```python
from build123d import *
from build123d.topology import SkipClean

# Parameters (mm, degrees)
SWEEP_2_DEPTH        = 3
SKETCH_15_W          = 3
SKETCH_15_H          = 8
SKETCH_17_W          = 3
SKETCH_17_H          = 8
REVOLVE_1_ANGLE      = 60
SKETCH_20_R          = 26.546275206
EXTRUDE_1_DEPTH      = 3
SKETCH_21_R          = 12.5
CUT_EXTRUDE_1_DEPTH  = 10
CUT_EXTRUDE_2_REACH  = 67.765
SKETCH_22_R          = 17
EXTRUDE_START        = 22
SKETCH_23_R          = 16.5
SKETCH_23_R_2        = 12.5
EXTRUDE_2_DEPTH      = 22
SKETCH_24_R          = 70.041464106
CUT_EXTRUDE_3_DEPTH  = 10
SKETCH_27_R          = 3
EXTRUDE_4_DEPTH      = 5
SKETCH_28_R          = 1.4
CUT_EXTRUDE_4_DEPTH  = 66.76473219
EXTRUDE_5_DEPTH      = 15
EXTRUDE_5_DEPTH_BACK = 3
SKETCH_30_R          = 1.4
EXTRUDE_6_DEPTH      = 3
EXTRUDE_9_DEPTH      = 8
SKETCH_34_R          = 1.5
CUT_EXTRUDE_5_DEPTH  = 13
SKETCH_35_R          = 57
SKETCH_35_R_2        = 37
CUT_EXTRUDE_6_DEPTH  = 69.556546004
FILLET_1_R           = 1
SKETCH_36_R          = 1.5
EXTRUDE_10_DEPTH     = 4
SKETCH_37_R          = 2
SKETCH_37_R_2        = 2.15
CUT_EXTRUDE_7_DEPTH  = 4


# Read off the part's stored shape, not the designer's step: 扫描2
with BuildPart() as part:
    # 扫描2 outline → 扫描2 (new body)
    with BuildSketch(Plane(origin=(0, 0, 0), x_dir=(1, 0, 0), z_dir=(0, 1, 0))):
        with BuildLine():
            ThreePointArc((-20, -34.641016151), (-12.679491924, -41.961524227), (-10, -51.961524227))
            Line((-10, -51.961524227), (11, -51.961524227))
            ThreePointArc((11, -51.961524227), (10.470745096, -45.395034193), (8.896644323, -38.998073283))
            ThreePointArc((8.896644323, -38.998073283), (5.963817028, 39.55291249), (-20, -34.641016151))
        make_face()
        with BuildLine():
            ThreePointArc((0, -24.015147002), (-4.46857992, -19.881209566), (-9.5, -16.454482672))
            ThreePointArc((-9.5, -16.454482672), (4.917561857, 18.352590699), (0, -19))
            Line((0, -19), (0, -24.015147002))
        make_face(mode=Mode.SUBTRACT)
    extrude(amount=SWEEP_2_DEPTH)

    # 扫描3: sweep along a path in 草图16
    with BuildLine(Plane(origin=(0, 3, 0), x_dir=(1, 0, 0), z_dir=(0, 1, 0))) as sweep_3_path:
        ThreePointArc((-10, -51.961524227), (-12.679491924, -41.961524227), (-20, -34.641016151))
        ThreePointArc((-20, -34.641016151), (5.963817027, 39.55291249), (8.896644323, -38.998073283))
    # 草图15 → 扫描3 (sweep)
    with BuildSketch(Plane.XY.offset(51.961524227)):
        with Locations((-8.5, 4)):
            Rectangle(SKETCH_15_W, SKETCH_15_H)
    sweep(path=sweep_3_path.line)

    # 草图17 → 旋转1 (revolve)
    with BuildSketch(Plane.XY.offset(51.961524227)):
        with Locations((12.5, 4)):
            Rectangle(SKETCH_17_W, SKETCH_17_H)
    revolve(axis=Axis((-30, 3, 51.961524227), (0, 1, 0)), revolution_arc=REVOLVE_1_ANGLE)

    # 草图20 → 凸台-拉伸1 (add)
    with BuildSketch(Plane(origin=(0, 3, 0), x_dir=(1, 0, 0), z_dir=(0, 1, 0))):
        Circle(SKETCH_20_R)
    extrude(amount=-EXTRUDE_1_DEPTH)

    # 草图21 → 切除-拉伸1 (cut)
    with BuildSketch(Plane(origin=(0, 3, 0), x_dir=(1, 0, 0), z_dir=(0, 1, 0))):
        with Locations(Location((0, 0, 0), (0, 0, 270))):
            Circle(SKETCH_21_R)
    extrude(amount=-CUT_EXTRUDE_1_DEPTH, mode=Mode.SUBTRACT)

    # 草图22 → 切除-拉伸2 (cut, up to next)
    with BuildSketch(Plane(origin=(0, 3, 0), x_dir=(1, 0, 0), z_dir=(0, 1, 0)), mode=Mode.PRIVATE) as cut_extrude_2_sk1:
        Circle(SKETCH_22_R)
    cut_extrude_2_tool1 = extrude(cut_extrude_2_sk1.sketch, amount=CUT_EXTRUDE_2_REACH, mode=Mode.PRIVATE) & part.part
    add(cut_extrude_2_tool1.solids().sort_by_distance((0, 3, 0))[0], mode=Mode.SUBTRACT)

    # 草图23 → 凸台-拉伸2 (add)
    with BuildSketch(Plane(origin=(0, 3, 0), x_dir=(1, 0, 0), z_dir=(0, 1, 0)).offset(EXTRUDE_START)):
        with Locations(Location((0, 0, 0), (0, 0, 270))):
            Circle(SKETCH_23_R)
        with Locations(Location((0, 0, 0), (0, 0, 270))):
            Circle(SKETCH_23_R_2, mode=Mode.SUBTRACT)
    extrude(amount=-EXTRUDE_2_DEPTH)

    # 草图24 → 切除-拉伸3 (cut)
    with BuildSketch(Plane(origin=(0, 3, 0), x_dir=(1, 0, 0), z_dir=(0, 1, 0))):
        Circle(SKETCH_24_R)
    extrude(amount=-CUT_EXTRUDE_3_DEPTH, mode=Mode.SUBTRACT)


with BuildPart() as cut_extrude_3_kept_piece:
    # of the separate pieces the step leaves, the one the design keeps (cut_extrude_3_pieces_kept)
    add(part.part.solids().sort_by_distance((-20, 8, 34.641016151))[0])

    # 草图27 → 凸台-拉伸4 (add)
    with BuildSketch(Plane(origin=(0, 8, 0), x_dir=(1, 0, 0), z_dir=(0, 1, 0))):
        with Locations((0, 40)):
            Circle(SKETCH_27_R)
        with Locations((34.641016151, 20)):
            Circle(SKETCH_27_R)
        with Locations((34.641016151, -20)):
            Circle(SKETCH_27_R)
        with Locations((-34.641016151, -20)):
            Circle(SKETCH_27_R)
        with Locations((-34.641016151, 20)):
            Circle(SKETCH_27_R)
    extrude(amount=-EXTRUDE_4_DEPTH)

    # 草图28 → 切除-拉伸4 (cut, through all)
    with BuildSketch(Plane(origin=(0, 8, 0), x_dir=(1, 0, 0), z_dir=(0, 1, 0))):
        with Locations(Location((0, 40, 0), (0, 0, 270))):
            Circle(SKETCH_28_R)
        with Locations(Location((34.641016151, 20, 0), (0, 0, 270))):
            Circle(SKETCH_28_R)
        with Locations(Location((34.641016151, -20, 0), (0, 0, 270))):
            Circle(SKETCH_28_R)
        with Locations((0, -40)):
            Circle(SKETCH_28_R)
        with Locations(Location((-34.641016151, -20, 0), (0, 0, 270))):
            Circle(SKETCH_28_R)
        with Locations(Location((-34.641016151, 20, 0), (0, 0, 270))):
            Circle(SKETCH_28_R)
    extrude(amount=-CUT_EXTRUDE_4_DEPTH, mode=Mode.SUBTRACT)

    # 草图30 → 凸台-拉伸5 (add, two sides: drawn at the far end of the back side and taken through both)
    # profile 1 of 2: a face of its own
    with BuildSketch(Plane(origin=(0, 8, 0), x_dir=(1, 0, 0), z_dir=(0, 1, 0)).offset(-EXTRUDE_5_DEPTH_BACK)):
        with BuildLine():
            ThreePointArc((-18.5, -32.04293994), (4.216428718, 36.758968006), (10.764012371, -35.399661547))
            Line((10.764012371, -35.399661547), (7.984647891, -36.528879457))
            ThreePointArc((7.984647891, -36.528879457), (10.239101404, -44.09929056), (11, -51.961524227))
            Line((11, -51.961524227), (14, -51.961524227))
            ThreePointArc((14, -51.961524227), (13.446319486, -45.003268476), (11.799212586, -38.220133207))
            ThreePointArc((11.799212586, -38.220133207), (23.753094696, -32.183699172), (33.044643352, -22.539998796))
            ThreePointArc((33.044643352, -22.539998796), (37.239092363, -21.5), (36.042533235, -17.347501204))
            ThreePointArc((36.042533235, -17.347501204), (40, 0), (36.042533235, 17.347501204))
            ThreePointArc((36.042533235, 17.347501204), (37.239092363, 21.5), (33.044643352, 22.539998796))
            ThreePointArc((33.044643352, 22.539998796), (20, 34.641016151), (2.997889883, 39.8875))
            ThreePointArc((2.997889883, 39.8875), (0, 43), (-2.997889883, 39.8875))
            ThreePointArc((-2.997889883, 39.8875), (-20, 34.641016151), (-33.044643352, 22.539998796))
            ThreePointArc((-33.044643352, 22.539998796), (-37.239092363, 21.5), (-36.042533235, 17.347501204))
            ThreePointArc((-36.042533235, 17.347501204), (-40, 0), (-36.042533235, -17.347501204))
            ThreePointArc((-36.042533235, -17.347501204), (-37.239092363, -21.5), (-33.044643352, -22.539998796))
            ThreePointArc((-33.044643352, -22.539998796), (-27.203716701, -29.325037044), (-20, -34.641016151))
            Line((-20, -34.641016151), (-18.5, -32.04293994))
        make_face()
        with Locations(Location((-34.641016151, -20, 0), (0, 0, 270))):
            Circle(SKETCH_30_R, mode=Mode.SUBTRACT)
        with Locations(Location((34.641016151, -20, 0), (0, 0, 270))):
            Circle(SKETCH_30_R, mode=Mode.SUBTRACT)
        with Locations(Location((-34.641016151, 20, 0), (0, 0, 270))):
            Circle(SKETCH_30_R, mode=Mode.SUBTRACT)
        with Locations(Location((0, 40, 0), (0, 0, 270))):
            Circle(SKETCH_30_R, mode=Mode.SUBTRACT)
        with Locations(Location((34.641016151, 20, 0), (0, 0, 270))):
            Circle(SKETCH_30_R, mode=Mode.SUBTRACT)
    # profile 2 of 2: a face of its own
    with BuildSketch(Plane(origin=(0, 8, 0), x_dir=(1, 0, 0), z_dir=(0, 1, 0)).offset(-EXTRUDE_5_DEPTH_BACK)):
        with BuildLine():
            Line((-20, -34.641016151), (-18.5, -32.04293994))
            ThreePointArc((-18.5, -32.04293994), (-10.081415713, -40.461524227), (-7, -51.961524227))
            Line((-7, -51.961524227), (-10, -51.961524227))
            ThreePointArc((-10, -51.961524227), (-12.679491924, -41.961524227), (-20, -34.641016151))
        make_face()
    extrude(amount=EXTRUDE_5_DEPTH + EXTRUDE_5_DEPTH_BACK)

    # 草图31 → 凸台-拉伸6 (add)
    with BuildSketch(Plane(origin=(0, 8, 0), x_dir=(1, 0, 0), z_dir=(0, 1, 0))):
        with BuildLine():
            Line((7.984647891, -36.528879457), (10.764012371, -35.399661547))
            ThreePointArc((10.764012371, -35.399661547), (4.742794362, -24.962667956), (-3.883880218, -16.550391973))
            ThreePointArc((-3.883880218, -16.550391973), (-6.259032022, -15.805838103), (-8.5, -14.722431864))
            Line((-8.5, -14.722431864), (-9.5, -16.454482672))
            ThreePointArc((-9.5, -16.454482672), (0.916967208, -25.033079439), (7.984647891, -36.528879457))
        make_face()
    extrude(amount=EXTRUDE_6_DEPTH)

    # 草图33 → 凸台-拉伸9 (add)
    with BuildSketch(Plane(origin=(0, 11, 0), x_dir=(1, 0, 0), z_dir=(0, 1, 0))):
        with BuildLine():
            Line((15.636875684, -33.53338812), (7.18451045, -15.40723238))
            ThreePointArc((7.18451045, -15.40723238), (1.746494616, -16.910048981), (-3.883880218, -16.550391973))
            ThreePointArc((-3.883880218, -16.550391973), (4.742794362, -24.962667956), (10.764012371, -35.399661547))
            ThreePointArc((10.764012371, -35.399661547), (13.23338455, -34.552532951), (15.636875684, -33.53338812))
        make_face()
    extrude(amount=-EXTRUDE_9_DEPTH)

    # 草图34 → 切除-拉伸5 (cut)
    with BuildSketch(Plane(origin=(0, 11, 0), x_dir=(1, 0, 0), z_dir=(0, 1, 0))):
        with Locations(Location((3.099042165, -20.843126869, 0), (0, 0, 270))):
            Circle(SKETCH_34_R)
        with Locations(Location((9.482973177, -29.801107938, 0), (0, 0, 270))):
            Circle(SKETCH_34_R)
    extrude(amount=-CUT_EXTRUDE_5_DEPTH, mode=Mode.SUBTRACT)

    # 草图35 → 切除-拉伸6 (cut, through all)
    with SkipClean():  # the faces are left unmerged after this step: merging them gives an invalid solid
        with BuildSketch(Plane.XZ.offset(-3)):
            Circle(SKETCH_35_R)
            Circle(SKETCH_35_R_2, mode=Mode.SUBTRACT)
        extrude(amount=-CUT_EXTRUDE_6_DEPTH, mode=Mode.SUBTRACT)

    # 圆角1
    fillet_1_edges = [cut_extrude_3_kept_piece.edges().sort_by_distance(p)[0] for p in [
        (15.636875684, 7, 33.53338812),
        (7.833230134, 7, 36.161312278),
        (7.18451045, 7, 15.40723238),
        (11.410693067, 11, 24.47031025),
        (0.786055573, 11, 24.883511334),
        (-9.5, 5.5, 16.454482672),
        (-8.5, 5.5, 14.722431864),
        (1.746494616, 11, 16.910048981),
    ]]
    fillet(fillet_1_edges, radius=FILLET_1_R - 0.0001)  # a hair under: the kernel refuses the full size

    # 草图36 → 凸台-拉伸10 (add)
    with BuildSketch(Plane(origin=(0, 11, 0), x_dir=(1, 0, 0), z_dir=(0, 1, 0))):
        with Locations(Location((9.482973177, -29.801107938, 0), (0, 0, 270))):
            Circle(SKETCH_36_R)
        with Locations(Location((3.099042165, -20.843126869, 0), (0, 0, 270))):
            Circle(SKETCH_36_R)
    extrude(amount=-EXTRUDE_10_DEPTH)

    # 草图37 → 切除-拉伸7 (cut)
    with BuildSketch(Plane.XZ.offset(-3)):
        with Locations(Location((3.099042165, 20.843126869, 0), (0, 0, 270))):
            Circle(SKETCH_37_R)
        with Locations(Location((9.482973177, 29.801107938, 0), (0, 0, 270))):
            Circle(SKETCH_37_R_2)
    extrude(amount=-CUT_EXTRUDE_7_DEPTH, mode=Mode.SUBTRACT)


solid = cut_extrude_3_kept_piece.part
```
Geometry check sheet. Reference: the model listing, model coordinates, mm. A direction names the side the tool comes from. Coordinates: 2 decimals unless noted, no trailing zeros. Answer as a JSON object with one key per item and string values.
Q1. Depth check by flat-ended pin: pin 1 Ø2.5 at (x, z) = (3.1, 20.84) entering from -Y. Enter the tip coordinate at first touch or a pass-through.
Results are:
{"pin 1": "stops at y = 7"}
Q2. Cross-section at A-A on y = 5.75. Give the number of separate pieces and of enclosed holes in the cut face, and give its area (3 significant figures).
Results are:
{"separate pieces": "1", "enclosed holes": "2", "area": "184 mm²"}
Q3. Tool access check on faces 4 (the cylindrical face through (10.13, 4.97, 27.75)), 5 (the cylindrical face through (12, 7, 35)). Record the directions out of +Z, -Z, +X, -X, +Y, -Y that give a thin tool (end or side, any length) a straight path to the whole face; none if there is none.
Results are:
{"face 4": "-Y", "face 5": "+Z, +X, +Y, -Y"}
Q4. Scan lines: line 1 (Z direction, x = 3, y = 6.5); line 2 (Y direction, x = 1.5, z = 21.25); line 3 (X direction, y = 3.5, z = 19.5). Record each from-to range of solid material in increasing order.
Results are:
{"line 1": "z = 16.73 to 18.85, 22.84 to 27.63", "line 2": "y = 7 to 11", "line 3": "x = -4.96 to 1.62, 4.58 to 9.09"}
Q5. Release check for a two-part mould opening along X. For faces 1 (the cylindrical face through (0.72, 6.45, 24.81)), 2 (the cylindrical face through (15.24, 6.94, 33.38)), 3 (the flat face through (3, 7, 21)) record: released by +X, released by -X, zero draft, split by the parting line, or undercut.
Results are:
{"face 1": "released by -X", "face 2": "released by +X", "face 3": "undercut"}
